Here's how the part is built. I have some questions about the finished solid (model axes, mm). A direction names the side the tool comes from. Round coordinates to 2 decimals unless told otherwise and drop trailing zeros. Order: outer loops, then holes, each group sorted by start corner. A loop starts at its lowest first (then second) coordinate and runs counter-clockwise, first axis right, second up. Notation, with made-up numbers: (6.5, 85.5) -> (18.5, 85.5) arc R29 ccw to (18.5, 118.5) -> close; hole circle Ø9 at (-38.75, 79). An arc over 180 degrees is marked (long way). Use a Markdown table: item, result. Add a question column.
(1) I want a section at A-A, the plane x = 10. Please give me the cut outline in (y, z), then the cut area to 3 significant figures.
(2) I want a section at C-C, the plane y = -7.5. Give the number of separate pieces and of enclosed holes in the cut face, then the cut area to 3 significant figures.
(3) If I drill on probe 1 along Z at (x, y) = (-15, -8); probe 2 along Z at (x, y) = (78, -6.75); probe 3 along X at (y, z) = (-8, -30), over which ranges is the centre line in solid material (lowest first)?
(4) On a 3-axis mill with a long thin cutter (end or side, diameter ignored), from which of +Z, -Z, +X, -X, +Y, -Y can I reach the whole of each face in a straight line? I mean faces 1 (the face through (-73.99, -5.07, 0.61)), 2 (the face through (30.005, -4.93, 7.5)). Say none if no direction works.
(5) I want a section at B-B, the plane z = -14. Please give me the cut outline in (x, y).
(6) I'm going to push flat-ended pins straight in: P1, Ø1, axis at y = -2, z = -25.5, coming from the -X side; P2, Ø9, axis at x = 10, z = 7.72, coming from the +Y side; P3, Ø3, axis at x = -101, y = -6.5, coming from the -Z side. Where does each tip first touch, or does it pass through?
(7) Thinking about a two-plate mould opening in X: for faces 3 (the face through (110, -5, 1)), 4 (the face through (-100, -5, -5.27)), 5 (the face through (83.96, -4.93, 28.62)), which applies, pulls with the +X half, pulls with the -X half, needs draft (parallel to the pull), parting line crosses it, or undercut?
from build123d import *

# Parameters (mm, degrees)
SKETCH1_W                    = 220
SKETCH1_H                    = 120
BOSS_EXTRUDE1_DEPTH          = 10
CUT_EXTRUDE1_REACH           = 127.698
SKETCH2_W                    = 20.632503002
SKETCH2_H                    = 54.730004003
F_12_5_12_5_DIAMETER_HOLE1_D = 12.5
F_10_0_10_DIAMETER_HOLE1_D   = 10
F_5_0MM_DOWEL_HOLE1_D        = 5
CUT_EXTRUDE2_REACH           = 127.698
SKETCH12_R                   = 4
SKETCH12_W                   = 81.05559148
SKETCH12_H                   = 15.93559148
SKETCH12_W_2                 = 21.30559148
SKETCH12_H_2                 = 20.21559148
SKETCH12_W_3                 = 21.55559148
DRAFT1_ANGLE                 = -1


with BuildPart() as part:
    # Sketch1 → Boss-Extrude1 (new body)
    with BuildSketch(Plane(origin=(0, 0, 0), x_dir=(1, 0, 0), z_dir=(0, 1, 0))):
        Rectangle(SKETCH1_W, SKETCH1_H)
    extrude(amount=-BOSS_EXTRUDE1_DEPTH)

    # Sketch2 → Cut-Extrude1 (cut, up to next)
    with BuildSketch(Plane(origin=(0, 0, 0), x_dir=(1, 0, 0), z_dir=(0, 1, 0)), mode=Mode.PRIVATE) as cut_extrude1_sk1:
        with Locations((-99.683748499, 32.634997999)):
            Rectangle(SKETCH2_W, SKETCH2_H)
    cut_extrude1_tool1 = extrude(cut_extrude1_sk1.sketch, amount=-CUT_EXTRUDE1_REACH, mode=Mode.PRIVATE) & part.part
    add(cut_extrude1_tool1.solids().sort_by_distance((-99.683748, 0, -32.634998))[0], mode=Mode.SUBTRACT)

    # Ø12.5 (12.5) Diameter Hole1 (through all)
    with Locations(Plane(origin=(0, -10, 0), x_dir=(-1, 0, 0), z_dir=(0, -1, 0))):
        with Locations((-98, 30), (-78, 30), (70, 30), (-98, -30.5), (-78, -30.5), (70, -27.22)):
            Hole(F_12_5_12_5_DIAMETER_HOLE1_D / 2)

    # Ø10.0 (10) Diameter Hole1 (through all)
    with Locations(Plane(origin=(0, -10, 0), x_dir=(-1, 0, 0), z_dir=(0, -1, 0))):
        with Locations((-60, -7.72), (-35, -7.72), (-10, -7.72), (15, -7.72)):
            Hole(F_10_0_10_DIAMETER_HOLE1_D / 2)

    # Ø5.0mm Dowel Hole1 (through all)
    with Locations(Plane(origin=(0, -10, 0), x_dir=(-1, 0, 0), z_dir=(0, -1, 0))):
        with Locations((30, -43.22), (55, -31.22)):
            Hole(F_5_0MM_DOWEL_HOLE1_D / 2)

    # Sketch12 → Cut-Extrude2 (cut, up to next)
    with BuildSketch(Plane.XZ.offset(10), mode=Mode.PRIVATE) as cut_extrude2_sk1:
        with Locations(Location((-90, 14.72, 0), (0, 0, 270))):
            Circle(SKETCH12_R)
    cut_extrude2_tool1 = extrude(cut_extrude2_sk1.sketch, amount=-CUT_EXTRUDE2_REACH, mode=Mode.PRIVATE) & part.part
    # Sketch12 → Cut-Extrude2 (cut, up to next)
    with BuildSketch(Plane.XZ.offset(10), mode=Mode.PRIVATE) as cut_extrude2_sk2:
        with Locations(Location((-70, -0.28, 0), (0, 0, 270))):
            Circle(SKETCH12_R)
    cut_extrude2_tool2 = extrude(cut_extrude2_sk2.sketch, amount=-CUT_EXTRUDE2_REACH, mode=Mode.PRIVATE) & part.part
    # Sketch12 → Cut-Extrude2 (cut, up to next)
    with BuildSketch(Plane.XZ.offset(10), mode=Mode.PRIVATE) as cut_extrude2_sk3:
        with Locations(Location((-50, 14.72, 0), (0, 0, 270))):
            Circle(SKETCH12_R)
    cut_extrude2_tool3 = extrude(cut_extrude2_sk3.sketch, amount=-CUT_EXTRUDE2_REACH, mode=Mode.PRIVATE) & part.part
    # Sketch12 → Cut-Extrude2 (cut, up to next)
    with BuildSketch(Plane.XZ.offset(10), mode=Mode.PRIVATE) as cut_extrude2_sk4:
        with Locations(Location((-30, -0.28, 0), (0, 0, 270))):
            Circle(SKETCH12_R)
    cut_extrude2_tool4 = extrude(cut_extrude2_sk4.sketch, amount=-CUT_EXTRUDE2_REACH, mode=Mode.PRIVATE) & part.part
    # Sketch12 → Cut-Extrude2 (cut, up to next)
    with BuildSketch(Plane.XZ.offset(10), mode=Mode.PRIVATE) as cut_extrude2_sk5:
        with Locations((20, 32.16)):
            Rectangle(SKETCH12_W, SKETCH12_H)
    cut_extrude2_tool5 = extrude(cut_extrude2_sk5.sketch, amount=-CUT_EXTRUDE2_REACH, mode=Mode.PRIVATE) & part.part
    # Sketch12 → Cut-Extrude2 (cut, up to next)
    with BuildSketch(Plane.XZ.offset(10), mode=Mode.PRIVATE) as cut_extrude2_sk6:
        with Locations((-9.875, -18.86)):
            Rectangle(SKETCH12_W_2, SKETCH12_H_2)
    cut_extrude2_tool6 = extrude(cut_extrude2_sk6.sketch, amount=-CUT_EXTRUDE2_REACH, mode=Mode.PRIVATE) & part.part
    # Sketch12 → Cut-Extrude2 (cut, up to next)
    with BuildSketch(Plane.XZ.offset(10), mode=Mode.PRIVATE) as cut_extrude2_sk7:
        with Locations((30, -18.86)):
            Rectangle(SKETCH12_W_3, SKETCH12_H_2)
    cut_extrude2_tool7 = extrude(cut_extrude2_sk7.sketch, amount=-CUT_EXTRUDE2_REACH, mode=Mode.PRIVATE) & part.part
    add(cut_extrude2_tool1.solids().sort_by_distance((-90, -10, 14.72))[0], mode=Mode.SUBTRACT)
    add(cut_extrude2_tool2.solids().sort_by_distance((-70, -10, -0.28))[0], mode=Mode.SUBTRACT)
    add(cut_extrude2_tool3.solids().sort_by_distance((-50, -10, 14.72))[0], mode=Mode.SUBTRACT)
    add(cut_extrude2_tool4.solids().sort_by_distance((-30, -10, -0.28))[0], mode=Mode.SUBTRACT)
    add(cut_extrude2_tool5.solids().sort_by_distance((20, -10, 32.16))[0], mode=Mode.SUBTRACT)
    add(cut_extrude2_tool6.solids().sort_by_distance((-9.875, -10, -18.86))[0], mode=Mode.SUBTRACT)
    add(cut_extrude2_tool7.solids().sort_by_distance((30, -10, -18.86))[0], mode=Mode.SUBTRACT)

    # Draft1
    draft1_faces = [part.faces().sort_by_distance(p)[0] for p in [
        (60.52779574, -5, 32.16),
        (20, -5, 40.12779574),
        (-20.52779574, -5, 32.16),
        (20, -5, 24.19220426),
        (-9.875, -5, -8.75220426),
        (30, -5, -8.75220426),
        (40.77779574, -5, -18.86),
        (0.77779574, -5, -18.86),
        (-20.52779574, -5, -18.86),
        (19.22220426, -5, -18.86),
        (30, -5, -28.96779574),
        (-9.875, -5, -28.96779574),
        (-50, -5, 18.72),
        (-30, -5, 3.72),
        (-70, -5, 3.72),
        (-90, -5, 18.72),
    ]]
    draft(draft1_faces, Plane.ZX, DRAFT1_ANGLE)


solid = part.part
Taken from the geometry:
| question | item | result |
|---|---|---|
| 1 | outline | (-10, -60) -> (0, -60) -> (0, 2.72) -> (-10, 2.72) -> close; (-10, 12.72) -> (0, 12.72) -> (0, 24.19) -> (-10, 24.02) -> close; (-10, 40.3) -> (0, 40.13) -> (0, 60) -> (-10, 60) -> close |
| 1 | area | 939 mm2 |
| 2 | separate pieces | 1 |
| 2 | enclosed holes | 19 |
| 2 | area | 21,800 mm2 |
| 3 | probe 1 | z = -60 to -29.11, -8.61 to 2.72, 12.72 to 24.05, 40.27 to 60 |
| 3 | probe 2 | z = -60 to -36.25, -23.75 to 24.25, 36.75 to 60 |
| 3 | probe 3 | x = -89.37 to -76.25, -63.75 to 71.75, 84.25 to 91.75, 104.25 to 110 |
| 4 | face 1 | -Y |
| 4 | face 2 | +Y, -Y |
| 5 | outline | (-89.37, -10) -> (-20.7, -10) -> (-20.53, 0) -> (-89.37, 0) -> close; (0.78, 0) -> (0.95, -10) -> (19.05, -10) -> (19.22, 0) -> close; (40.78, 0) -> (40.95, -10) -> (110, -10) -> (110, 0) -> close |
| 6 | P1 | stops at x = -89.37 |
| 6 | P2 | passes through |
| 6 | P3 | stops at z = -5.27 |
| 7 | face 3 | pulls with the +X half |
| 7 | face 4 | needs draft |
| 7 | face 5 | undercut |
